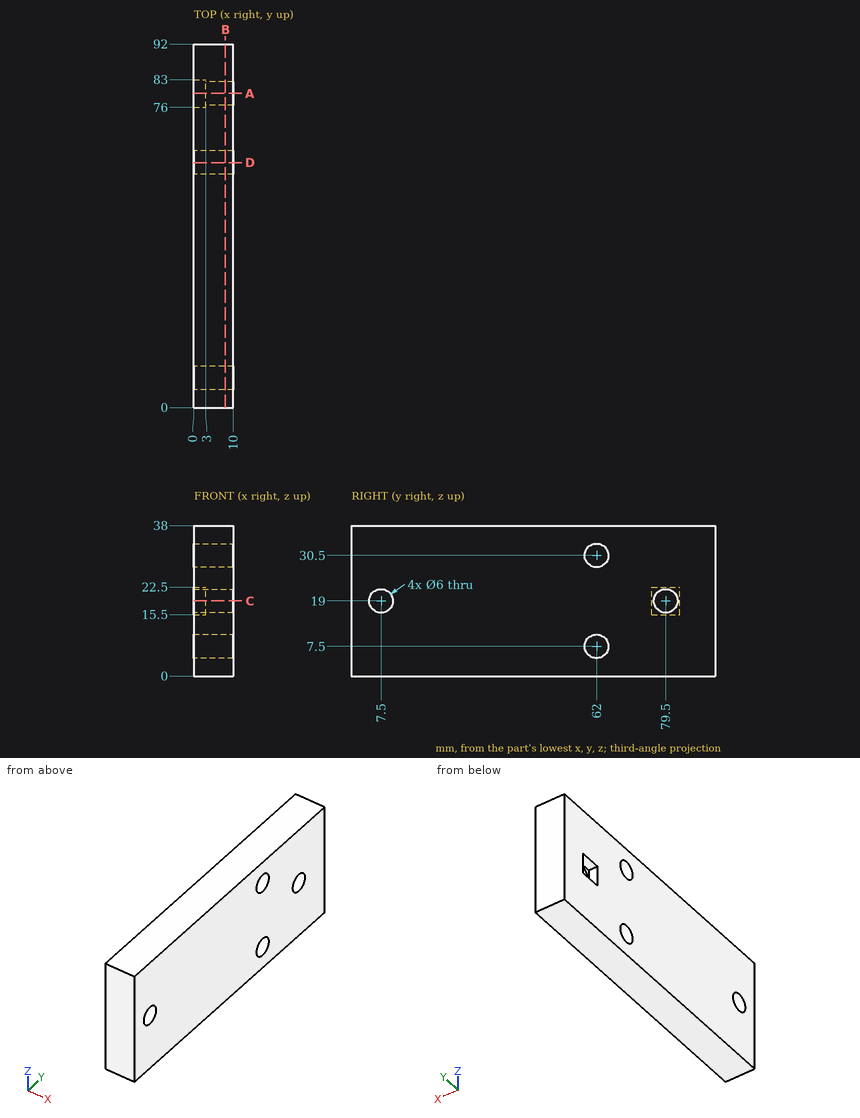
For this review, use the dimensioned drawing (mm, ordinates from the lowest corner) and the shaded views. Give positions to 0.01 mm unless a question says otherwise; leave off trailing zeros. Order: outer loops, then holes, each group sorted by start corner. A loop starts at its lowest first (then second) coordinate and runs counter-clockwise, first axis right, second up. Notation, with made-up numbers: (65.25, 69) -> (120.25, 69) arc R19 cw to (120.25, 76) -> close; hole circle Ø8 at (79, 89). An arc over 180 degrees is marked (long way). Write item = value, one per line. Start each with the question number.
(1) Take a section at B-B (x = 8). Write out the cut boundary in (y, z), plus the area to 3 significant figures.
(2) Take a section at A-A (y = 79.5). Write out the cut boundary in (x, z).
(3) Take a section at D-D (y = 62). Write out the cut boundary in (x, z), plus the area to 3 significant figures.
(4) For L1, parallel to Y at x = 6, z = 19; L2, parallel to Y at x = 3.5, z = 21.5; L3, parallel to Z at x = 3.25, y = 64, list the stretches that pass through material, from the lowest coordinate up. Write a range as from..to.
(5) Take a section at C-C (z = 19). Write out the cut boundary in (x, y).
Returned:
q1.outline = (0, 0) -> (92, 0) -> (92, 38) -> (0, 38) -> close; hole circle Ø6 at (7.5, 19); hole circle Ø6 at (62, 7.5); hole circle Ø6 at (62, 30.5); hole circle Ø6 at (79.5, 19)
q1.area = 3,380 mm²
q2.outline = (0, 0) -> (10, 0) -> (10, 16) -> (3, 16) -> (3, 15.5) -> (0, 15.5) -> close; (0, 22.5) -> (3, 22.5) -> (3, 22) -> (10, 22) -> (10, 38) -> (0, 38) -> close
q3.outline = (0, 0) -> (10, 0) -> (10, 4.5) -> (0, 4.5) -> close; (0, 10.5) -> (10, 10.5) -> (10, 27.5) -> (0, 27.5) -> close; (0, 33.5) -> (10, 33.5) -> (10, 38) -> (0, 38) -> close
q3.area = 260 mm²
q4.L1 = 0..4.5, 10.5..76.5, 82.5..92
q4.L2 = 0..5.84, 9.16..77.84, 81.16..92
q4.L3 = 0..5.26, 9.74..28.26, 32.74..38
q5.outline = (0, 0) -> (10, 0) -> (10, 4.5) -> (0, 4.5) -> close; (0, 10.5) -> (10, 10.5) -> (10, 76.5) -> (3, 76.5) -> (3, 76) -> (0, 76) -> close; (0, 83) -> (3, 83) -> (3, 82.5) -> (10, 82.5) -> (10, 92) -> (0, 92) -> close
